from build123d import *

# Parameters (mm, degrees)
BASE_DEPTH                      = 6
SKETCH2_R                       = 5.5
SHAFT_HOLDING_BODY_DEPTH        = 12
M4X0_7_TAPPED_HOLE1_D           = 3.3
M4X0_7_TAPPED_HOLE1_CSINK_D     = 4
M4X0_7_TAPPED_HOLE1_CSINK_ANGLE = 90
M3X0_5_TAPPED_HOLE1_D           = 2.5
SKETCH13_R                      = 3
SHAFT_HOLE_DEPTH                = 13.5
SH_C_SIZE                       = 0.2


with BuildPart() as part:
    # Sketch1 → BASE (new body)
    with BuildSketch(Plane(origin=(0, 0, 0), x_dir=(1, 0, 0), z_dir=(0, 1, 0))):
        Polygon((3.464101615, -6), (6.92820323, 0), (3.464101615, 6), (-3.464101615, 6), (-6.92820323, 0), (-3.464101615, -6), align=None)
    extrude(amount=BASE_DEPTH)

    # Sketch2 → SHAFT HOLDING BODY (add)
    with BuildSketch(Plane(origin=(0, 6, 0), x_dir=(1, 0, 0), z_dir=(0, 1, 0))):
        with Locations(Location((0, 0, 0), (0, 0, 270))):
            Circle(SKETCH2_R)
    extrude(amount=SHAFT_HOLDING_BODY_DEPTH)

    # M4x0.7 Tapped Hole1 (through all)
    with Locations(Plane(origin=(0, 0, 0), x_dir=(-1, 0, 0), z_dir=(0, -1, 0))):
        with Locations((0, 0)):
            CounterSinkHole(M4X0_7_TAPPED_HOLE1_D / 2, M4X0_7_TAPPED_HOLE1_CSINK_D / 2, counter_sink_angle=M4X0_7_TAPPED_HOLE1_CSINK_ANGLE)

    # M3x0.5 Tapped Hole1 (through all)
    with Locations(Plane(origin=(2.75, 6, 4.763139721), x_dir=(0.8660254037844385, 0, -0.5000000000000004), z_dir=(0.5000000000000003, 0, 0.8660254037844384))):
        with Locations((0, 9)):
            Hole(M3X0_5_TAPPED_HOLE1_D / 2)

    # Sketch9 → BASE CHAMFER RELIEF (revolve, cut)
    with BuildSketch(Plane.XY, mode=Mode.PRIVATE) as base_chamfer_relief_sk:
        with BuildLine():
            Line((-6.92820323, 1), (-6.92820323, 0))
            Line((-6.92820323, 0), (-5.92820323, 0))
            ThreePointArc((-5.92820323, 0), (-6.635310011, 0.292893219), (-6.92820323, 1))
        make_face()
    revolve(base_chamfer_relief_sk.sketch.rotate(Axis((0, 0, 0), (0, -1, 0)), 90), axis=Axis((0, 0, 0), (0, -1, 0)), mode=Mode.SUBTRACT)

    # Sketch13 → SHAFT HOLE (cut)
    with BuildSketch(Plane(origin=(0, 18, 0), x_dir=(1, 0, 0), z_dir=(0, 1, 0))):
        with Locations(Location((0, 0, 0), (0, 0, 270))):
            Circle(SKETCH13_R)
    extrude(amount=-SHAFT_HOLE_DEPTH, mode=Mode.SUBTRACT)

    # SH C
    sh_c_edges = [part.edges().sort_by_distance(p)[0] for p in [
        (0, 18, -3),
    ]]
    chamfer(sh_c_edges, length=SH_C_SIZE)


solid = part.part
Verification items for the finished model (mm, model axes). A direction names the side the tool comes from. Round coordinates to 2 decimals unless told otherwise and drop trailing zeros. Loops run counter-clockwise (first coordinate to the right, second up) from the corner with the lowest first, then second, coordinate; pieces in that order, holes last. Notation, with made-up numbers: (-40, 59.5) - (-17, 59.5) arc R15 cw to (-17, 78.5) - close; hole circle Ø5 at (63, -1). An arc over 180 degrees is marked (long way). Answer in a Markdown table with one row per item. Add a question column.
Q1. Section check A-A on x = 0. Enter the section's corners in (y, z).
Q2. Tool access check on faces 4 (the face through (5.22, 2.96, -2.96)), 5 (the face through (5, 6, -3)). Record the directions out of +Z, -Z, +X, -X, +Y, -Y that give a thin tool (end or side, any length) a straight path to the whole face; none if there is none.
Q3. Section check B-B on y = 11.75. Enter the section's corners in (x, z).
Q4. Material ranges on line 1 (Z direction, x = 0, y = 3.4); line 2 (X direction, y = 17.75, z = -2.75); line 3 (Y direction, x = -4.75, z = 3), recorded low to high.
Q5. Release check for a two-part mould opening along Z. For faces 1 (the face through (5.172, 2.959, 3.042)), 2 (the face through (-1.21, 14.24, -4.08)), 3 (the face through (3, 0, 0)) record: pulls with the +Z half, pulls with the -Z half, needs draft (parallel to the pull), parting line crosses it, or undercut.
Q6. Gauge pin test, flat ends, axial feed: pin 1 (1.5 mm diameter, centred on x = 4.5, y = 13, fed in from +Z); pin 2 (2 mm diameter, centred on x = 5, z = 4, fed in from -Y); pin 3 (1.8 mm diameter, centred on x = 0.5, z = -1, fed in from +Y); pin 4 (3 mm diameter, centred on y = 8.5, z = -0.5, fed in from +X). Record the tip position at first contact, or that the pin passes through.
Found:
| question | item | result |
|---|---|---|
| 1 | outline | (0, -6) - (6, -6) - (6, -5.5) - (18, -5.5) - (18, -3.2) - (17.8, -3) - (4.5, -3) - (4.5, -1.65) - (0.35, -1.65) - (0, -2) - (0, -5.93) arc R1 ccw to start; (0, 2) - (0.35, 1.65) - (4.5, 1.65) - (4.5, 3) - (17.8, 3) - (18, 3.2) - (18, 5.5) - (6, 5.5) - (6, 6) - (0, 6) arc R1 ccw to (0, 5.93) - close |
| 2 | face 4 | -Z, +X, +Y, -Y |
| 2 | face 5 | +Y |
| 3 | outline | circle Ø11 at (0, 0); hole circle Ø6 at (0, 0) |
| 4 | line 1 | z = -6 to -1.65, 1.65 to 6 |
| 4 | line 2 | x = -4.76 to -1.2, 1.2 to 4.76 |
| 4 | line 3 | y = 0 to 6 |
| 5 | face 1 | pulls with the +Z half |
| 5 | face 2 | undercut |
| 5 | face 3 | needs draft |
| 6 | pin 1 | stops at z = 4.02 |
| 6 | pin 2 | stops at y = 0 |
| 6 | pin 3 | stops at y = 4.5 |
| 6 | pin 4 | stops at x = 5.5 |
